```python
from build123d import *

# Parameters (mm, degrees)
SKETCH_1_W      = 77
SKETCH_1_H      = 136
SKETCH_1_R      = 1.55
SKETCH_1_R_2    = 1.05
SKETCH_1_W_2    = 24
SKETCH_1_H_2    = 2
EXTRUDE_1_DEPTH = 2


with BuildPart() as part:
    # 草图1 → 凸台-拉伸1 (new body)
    with BuildSketch(Plane(origin=(0, 0, 0), x_dir=(1, 0, 0), z_dir=(0, 1, 0))):
        with Locations((38.5, 68)):
            Rectangle(SKETCH_1_W, SKETCH_1_H)
        with Locations(Location((7.71, 72.38, 0), (0, 0, 270))):
            Circle(SKETCH_1_R, mode=Mode.SUBTRACT)
        with Locations(Location((6.71, 10.34, 0), (0, 0, 270))):
            Circle(SKETCH_1_R, mode=Mode.SUBTRACT)
        with Locations(Location((63.71, 71.44, 0), (0, 0, 270))):
            Circle(SKETCH_1_R, mode=Mode.SUBTRACT)
        with Locations(Location((64.31, 37.24, 0), (0, 0, 270))):
            Circle(SKETCH_1_R, mode=Mode.SUBTRACT)
        with Locations(Location((21.81, 21.74, 0), (0, 0, 270))):
            Circle(SKETCH_1_R, mode=Mode.SUBTRACT)
        with Locations(Location((55.01, 21.74, 0), (0, 0, 270))):
            Circle(SKETCH_1_R, mode=Mode.SUBTRACT)
        with Locations(Location((21.81, 59.84, 0), (0, 0, 270))):
            Circle(SKETCH_1_R, mode=Mode.SUBTRACT)
        with Locations(Location((55.01, 59.84, 0), (0, 0, 270))):
            Circle(SKETCH_1_R, mode=Mode.SUBTRACT)
        with Locations(Location((6.5, 127.4, 0), (0, 0, 270))):
            Circle(SKETCH_1_R_2, mode=Mode.SUBTRACT)
        with Locations(Location((30.5, 127.4, 0), (0, 0, 270))):
            Circle(SKETCH_1_R_2, mode=Mode.SUBTRACT)
        with Locations(Location((6.3, 83.8, 0), (0, 0, 270))):
            Circle(SKETCH_1_R_2, mode=Mode.SUBTRACT)
        with Locations(Location((30.7, 83.8, 0), (0, 0, 270))):
            Circle(SKETCH_1_R_2, mode=Mode.SUBTRACT)
        with Locations(Location((38.5, 124, 0), (0, 0, 270))):
            Circle(SKETCH_1_R_2, mode=Mode.SUBTRACT)
        with Locations(Location((63.9, 124, 0), (0, 0, 270))):
            Circle(SKETCH_1_R_2, mode=Mode.SUBTRACT)
        with Locations(Location((38.5, 83, 0), (0, 0, 270))):
            Circle(SKETCH_1_R_2, mode=Mode.SUBTRACT)
        with Locations(Location((63.9, 83, 0), (0, 0, 270))):
            Circle(SKETCH_1_R_2, mode=Mode.SUBTRACT)
        with Locations(Location((3, 3, 0), (0, 0, 270))):
            Circle(SKETCH_1_R_2, mode=Mode.SUBTRACT)
        with Locations(Location((75, 3, 0), (0, 0, 270))):
            Circle(SKETCH_1_R_2, mode=Mode.SUBTRACT)
        with Locations(Location((3, 133, 0), (0, 0, 270))):
            Circle(SKETCH_1_R_2, mode=Mode.SUBTRACT)
        with Locations(Location((74, 133, 0), (0, 0, 270))):
            Circle(SKETCH_1_R_2, mode=Mode.SUBTRACT)
        with BuildLine():
            Line((53, 65.2), (53, 55))
            ThreePointArc((53, 55), (50.5, 52.5), (48, 55))
            Line((48, 55), (48, 65.2))
            ThreePointArc((48, 65.2), (50.5, 67.7), (53, 65.2))
        make_face(mode=Mode.SUBTRACT)
        with Locations((35, 2.5)):
            Rectangle(SKETCH_1_W_2, SKETCH_1_H_2, mode=Mode.SUBTRACT)
    extrude(amount=EXTRUDE_1_DEPTH)


solid = part.part
```
CAD build for the part. Positions are in the model's coordinates, mm. A direction names the side the tool comes from. Round coordinates to 2 decimals unless told otherwise and drop trailing zeros. Write each loop counter-clockwise with the first axis right and the second up, starting at its lowest first coordinate (ties: lowest second). Pieces come first, ordered by that corner, then holes.
Item 1: Drill centre lines: L1, parallel to X at y = 0.45, z = -59.84; L2, parallel to X at y = 1.4, z = -3; L3, parallel to X at y = 1.55, z = -133. Where is each one in solid material? Low to high.
Filled in:
L1: x = 0 to 20.26, 23.36 to 48, 53 to 53.46, 56.56 to 77
L2: x = 0 to 1.95, 4.05 to 23, 47 to 73.95, 76.05 to 77
L3: x = 0 to 1.95, 4.05 to 72.95, 75.05 to 77
Item 2: Drop a flat-ended pin along its axis: pin 1 Ø3 at (x, z) = (55.01, -59.84) entering from +Y. Give the stop position or say it passes through.
Filled in:
pin 1: passes through
Item 3: Tool access for faces 3 (the flat face through (38, 0, -69)), 4 (the cylindrical face through (50.6, 1, -52.5)): list every direction of +Z, -Z, +X, -X, +Y, -Y with a clear straight run to the whole face (end or side of a thin tool).
Filled in:
face 3: +Z, -Z, +X, -X, -Y
face 4: +Y, -Y
Item 4: Mould opens along X. For faces 1 (the flat face through (38, 2, -69)), 2 (the cylindrical face through (7.76, 0.99, -11.48)) say: released by +X, released by -X, zero draft, split by the parting line, or undercut.
Filled in:
face 1: zero draft
face 2: undercut
Item 5: Band-saw the part on A-A on x = 55.01. Write the cut outline in (y, z).
Filled in:
outline: (0, -136) - (2, -136) - (2, -61.39) - (0, -61.39) - close; (0, -58.29) - (2, -58.29) - (2, -23.29) - (0, -23.29) - close; (0, -20.19) - (2, -20.19) - (2, 0) - (0, 0) - close
Item 6: Band-saw the part on B-B on y = 0.6. Give the number of separate pieces and of enclosed holes in the cut face, then the cut area to 3 significant figures.
Filled in:
separate pieces: 1
enclosed holes: 22
area: 10,300 mm2
